The figure shows three views and two pictorial views of one solid part (mm, origin at its lowest corner). Answer the questions. A direction names the side the tool comes from. Round coordinates to 2 decimals unless told otherwise and drop trailing zeros. Order: outer loops, then holes, each group sorted by start corner. A loop starts at its lowest first (then second) coordinate and runs counter-clockwise, first axis right, second up. Notation, with made-up numbers: (-19, -2) -> (39, -2) arc R27 ccw to (39, 31) -> close; hole circle Ø7 at (69.25, 40.5). An arc over 180 degrees is marked (long way). One line per item, written item: value. Start each with the question number.
1. Section D-D (x = 47) is taken. Give the vertices of the cut face in (y, z), then the cut area to 3 significant figures.
2. Section C-C (y = 10.5) is taken. Give the vertices of the cut face in (x, z), then the cut area to 3 significant figures.
3. Section A-A (z = 45.5) is taken. Give the vertices of the cut face in (x, y).
4. For the marked faces 1, 2 and 3, determine the directions among +Z, -Z, +X, -X, +Y, -Y from which every point of the face is accessible in a straight line to the end or side of a thin tool.
5. Flat-ended cylindrical pins translate along their axes: pin 1 Ø7 at (y, z) = (4, 46.5) entering from +X; pin 2 Ø4 at (x, y) = (37.5, 45) entering from +Z; pin 3 Ø5 at (y, z) = (49.5, 48) entering from -X; pin 4 Ø7.5 at (x, z) = (38.1, 12.7) entering from +Y. Find the tip coordinate at first contact, or state that the pin passes through.
6. Section B-B (x = 38.1) is taken. Give the vertices of the cut face in (y, z), then the cut area to 3 significant figures.
7. The mould has two halves that part along X. Classify the marked faces 4, 5 and 6: released by +X, released by -X, zero draft, split by the parting line, or undercut.
8. Consider line 1 (Z direction, x = 38, y = 14); line 2 (Z direction, x = 25.5, y = 16); line 3 (Z direction, x = 67.5, y = 5.5). Determine where each line is inside the solid, lowest interval first.
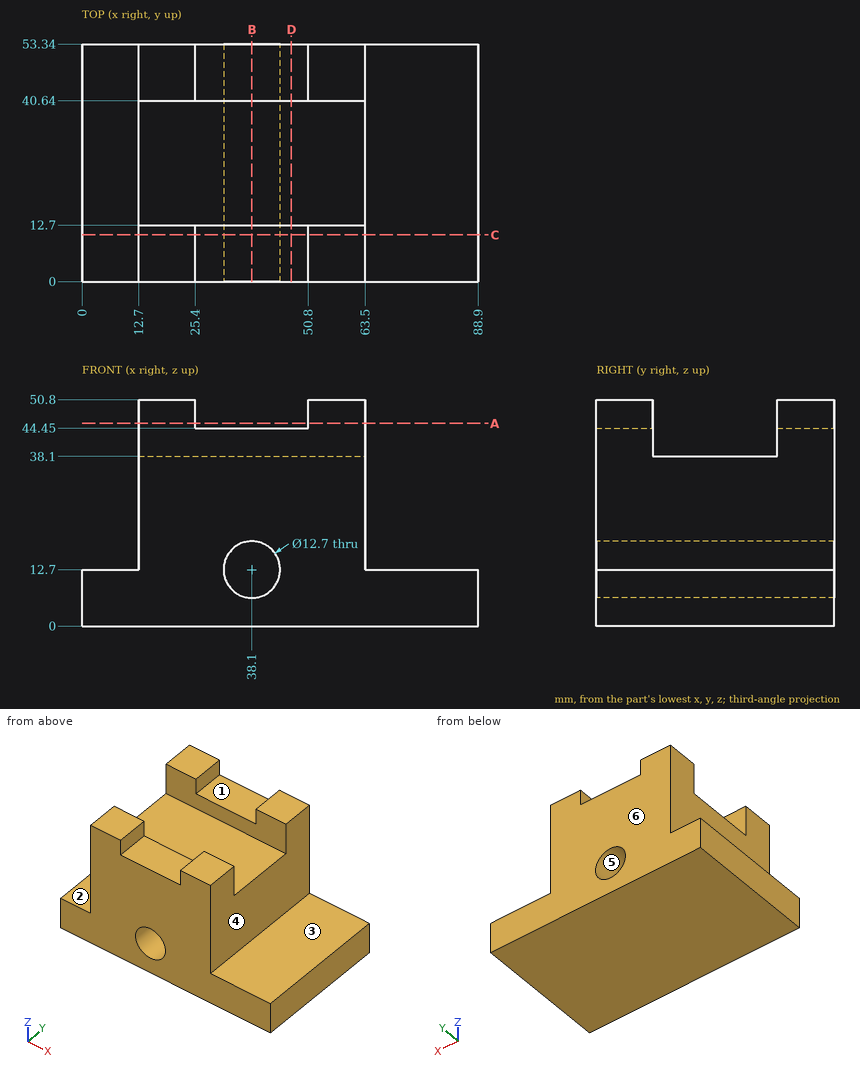
Answer:
1. outline: (0, 0) -> (53.34, 0) -> (53.34, 44.45) -> (40.64, 44.45) -> (40.64, 38.1) -> (12.7, 38.1) -> (12.7, 44.45) -> (0, 44.45) -> close
1. area: 2,190 mm^2
2. outline: (0, 0) -> (88.9, 0) -> (88.9, 12.7) -> (63.5, 12.7) -> (63.5, 50.8) -> (50.8, 50.8) -> (50.8, 44.45) -> (25.4, 44.45) -> (25.4, 50.8) -> (12.7, 50.8) -> (12.7, 12.7) -> (0, 12.7) -> close; hole circle Ø12.7 at (38.1, 12.7)
2. area: 2,780 mm^2
3. outline: (12.7, 0) -> (25.4, 0) -> (25.4, 12.7) -> (12.7, 12.7) -> close; (12.7, 40.64) -> (25.4, 40.64) -> (25.4, 53.34) -> (12.7, 53.34) -> close; (50.8, 0) -> (63.5, 0) -> (63.5, 12.7) -> (50.8, 12.7) -> close; (50.8, 40.64) -> (63.5, 40.64) -> (63.5, 53.34) -> (50.8, 53.34) -> close
4. face 1: +Z, +Y, -Y
4. face 2: +Z, -X, +Y, -Y
4. face 3: +Z, +X, +Y, -Y
5. pin 1: x = 63.5
5. pin 2: z = 44.45
5. pin 3: x = 12.7
5. pin 4: through
6. outline: (0, 0) -> (53.34, 0) -> (53.34, 6.35) -> (0, 6.35) -> close; (0, 19.05) -> (53.34, 19.05) -> (53.34, 44.45) -> (40.64, 44.45) -> (40.64, 38.1) -> (12.7, 38.1) -> (12.7, 44.45) -> (0, 44.45) -> close
6. area: 1,520 mm^2
7. face 4: released by +X
7. face 5: undercut
7. face 6: zero draft
8. line 1: 0 to 6.35, 19.05 to 38.1
8. line 2: 0 to 38.1
8. line 3: 0 to 12.7
